Check sheet for the modelled part. Datum: model origin and axes. Units: mm. Give positions to 0.01 mm unless a question says otherwise; leave off trailing zeros. Write each loop counter-clockwise with the first axis right and the second up, starting at its lowest first coordinate (ties: lowest second). Pieces come first, ordered by that corner, then holes. Notation, with made-up numbers: M -10.5,26.5 L 9.5,26.5 A25 cw 9.5,43.5 Z; hole C 53.25,80 d11. An arc over 180 degrees is marked long. Write item = value, one per line. Start each with the question number.
1) Cross-section at D-D, the plane x = 124. Record the cut outline in (y, z), plus the area to 3 significant figures.
2) Cross-section at C-C, the plane x = 17.5. Record the cut outline in (y, z).
3) Cross-section at A-A, the plane z = 2. Record the cut outline in (x, y).
4) Cross-section at B-B, the plane y = -15.75. Record the cut outline in (x, z).
5) Scan lines: line 1 along X through (y, z) = (-28.25, -20); line 2 along X through (y, z) = (-13.5, -13.5); line 3 along Z through (x, y) = (111, -8.5). Record each from-to range of solid material in increasing order. Write a range as [from, to].
6) Go/stop test with flat-tipped pins: pin 1 (1.5 mm diameter, centred on y = -14.5, z = -15.5, fed in from +X); pin 2 (8 mm diameter, centred on y = -6, z = -13.5, fed in from -X); pin 3 (10 mm diameter, centred on y = -16.5, z = 2, fed in from +X). Record where each tip stops, or that it passes through.
7) Mould release check, pull along X, two halves, no side actions. Record for faces 1 (the cylindrical face through (120, -15, 0)), 2 (the flat face through (241.064, -14.79, -15.21)), 3 (the flat face through (118, -15, -30)): released by +X, released by -X, zero draft, split by the parting line, or undercut.
```python
from build123d import *

# Parameters (mm, degrees)
F1_DEPTH = 30
F2_R     = 10
F3_DEPTH = 30


with BuildPart() as f1:
    # F0 (on Front) → F1 (new body)
    with BuildSketch(Plane.XZ):
        Polygon((120, 10), (0, 0), (240, 0), align=None)
        Polygon((240, 0), (0, 0), (-2.097804, -30), (120, -30), (242.097804, -30), align=None)
    extrude(amount=F1_DEPTH)

    # F2 (on face) → F3 (cut)
    with BuildSketch(Plane.XZ.offset(30)):
        with Locations((120, 10)):
            Circle(F2_R)
    extrude(amount=-F3_DEPTH, mode=Mode.SUBTRACT)


solid = f1.part
```
Reply:
q1.outline = M -30,-30 L 0,-30 L 0,0.83 L -30,0.83 Z
q1.area = 925 mm2
q2.outline = M -30,-30 L 0,-30 L 0,1.46 L -30,1.46 Z
q3.outline = M 24,-30 L 114,-30 L 114,0 L 24,0 Z; M 126,-30 L 216,-30 L 216,0 L 126,0 Z
q4.outline = M -2.1,-30 L 242.1,-30 L 240,0 L 129.97,9.17 A10 cw 110.03,9.17 L 0,0 Z
q5.line_1 = [-1.4, 241.4]
q5.line_2 = [-0.94, 240.94]
q5.line_3 = [-30, 5.64]
q6.pin_1 = 241.14
q6.pin_2 = -1.22
q6.pin_3 = 240.21
q7.face_1 = undercut
q7.face_2 = released by +X
q7.face_3 = zero draft
